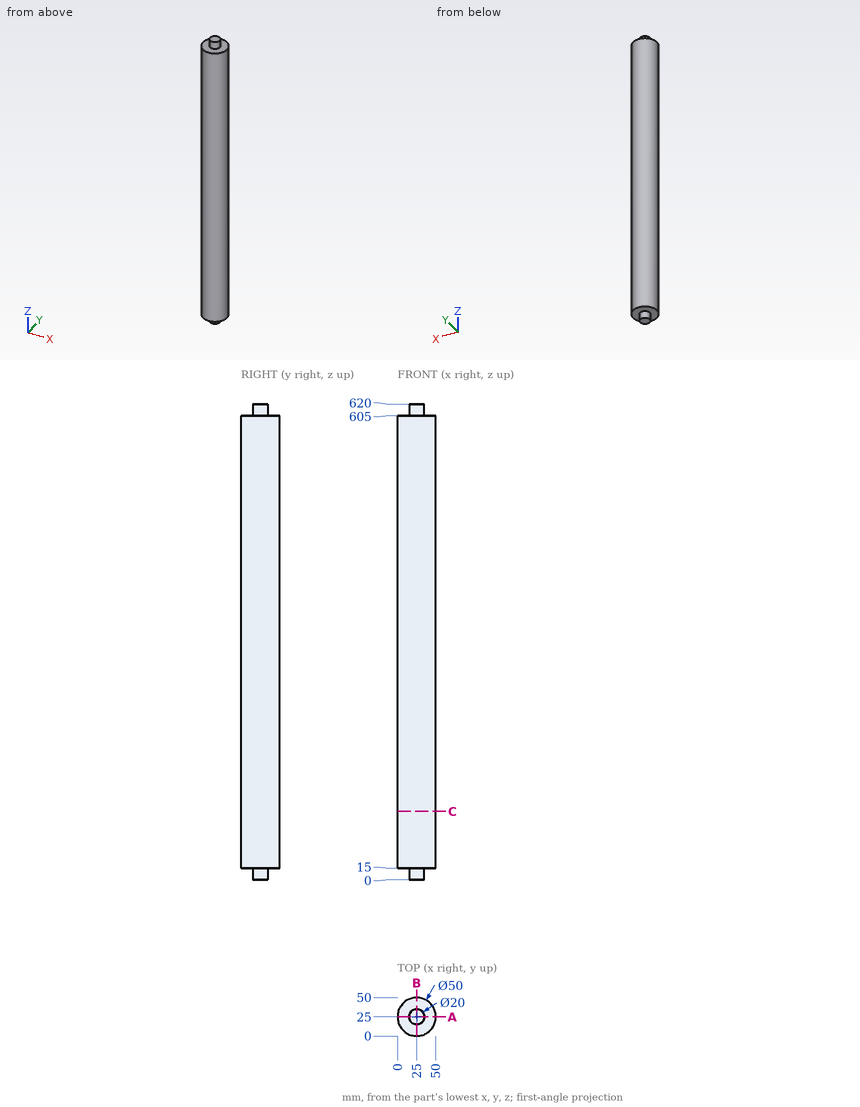
Geometry: see drawing. Coordinates: mm, zero at the bounding-box minimum. Give positions to 0.01 mm unless a question says otherwise; leave off trailing zeros. Order: outer loops, then holes, each group sorted by start corner. A loop starts at its lowest first (then second) coordinate and runs counter-clockwise, first axis right, second up. Notation, with made-up numbers: (86.25, -25.5) -> (102.25, -25.5) arc R22 cw to (102.25, -13.5) -> close; hole circle Ø11 at (65.25, 86). An arc over 180 degrees is marked (long way). Write each question's results on one line, items separated by ' | '. Start each with the question number.
1) Line query: line 1 (Y direction, x = 25, z = 539); line 2 (Z direction, x = 46, y = 16); line 3 (X direction, y = 26.5, z = 326). Output: solid intervals per line, ascending. Write a range as from..to.
2) Section C-C (z = 89). Return loops of the section in (x, y).
3) Section A-A (y = 25). Return loops of the section in (x, z), then the cut area to 3 significant figures.
4) First-contact query: pin 1 (2 mm diameter, centred on y = 9, z = 387.5, fed in from -X); pin 2 (2 mm diameter, centred on y = 6, z = 242, fed in from +X); pin 3 (1 mm diameter, centred on x = 10, z = 186, fed in from +Y). Flat tips, straight axial feed; report the tip coordinate or a pass-through.
Calculated:
1) line 1: 0..50 | line 2: 15..605 | line 3: 0.05..49.95
2) outline: circle Ø50 at (25, 25)
3) outline: (0, 15) -> (15, 15) -> (15, 0) -> (35, 0) -> (35, 15) -> (50, 15) -> (50, 605) -> (35, 605) -> (35, 620) -> (15, 620) -> (15, 605) -> (0, 605) -> close | area: 30,100 mm2
4) pin 1: x = 5 | pin 2: x = 42.35 | pin 3: y = 45.37
